Autodesk Inventor part; units mm, degrees
ref_plane "YZ Plane" through (0, 0, 0) normal (1, 0, 0) x (0, 1, 0)
ref_plane "XZ Plane" through (0, 0, 0) normal (0, 1, 0) x (-1, 0, 0)
ref_plane "XY Plane" through (0, 0, 0) normal (0, 0, 1) x (1, 0, 0)
sketch "Sketch1" plane through (0, 0, 0) normal (0, 1, 0) x (-1, 0, 0)
  line L0 (-19.05, 19.05) -> (19.05, 19.05)
  line L1 (19.05, 19.05) -> (19.05, -19.05)
  line L2 (19.05, -19.05) -> (-19.05, -19.05)
  line L3 (-19.05, -19.05) -> (-19.05, 19.05)
  circle A0 centre (0, 0) radius 6.35
  circle A1 centre (0, 0) radius 19.05 construction
  circle A2 centre (0, 0) radius 9.779 construction
  line L4 (19.05, -19.05) -> (-19.05, 19.05) construction
  line L5 (19.05, 19.05) -> (-19.05, -19.05) construction
  circle A3 centre (0, -9.779) radius 1.778
  circle A4 centre (6.9148, -6.9148) radius 1.778
  circle A5 centre (-6.9148, -6.9148) radius 1.778
  circle A6 centre (-6.9148, 6.9148) radius 1.778
  circle A7 centre (0, 9.779) radius 1.778
  circle A8 centre (6.9148, 6.9148) radius 1.778
  circle A9 centre (-9.779, 0) radius 2.032
  circle A10 centre (9.779, 0) radius 2.032
  circle A11 centre (-13.4704, 13.4704) radius 1.778
  circle A12 centre (13.4704, 13.4704) radius 1.778
  circle A13 centre (13.4704, -13.4704) radius 1.778
  circle A14 centre (-13.4704, -13.4704) radius 1.778
  dimension "d5" = 19.558
  dimension "d0" = 19.05
  dimension "d1" = 38.1
  dimension "d2" = 38.1
  dimension "d3" = 19.05
  dimension "d4" = 12.7
  dimension "d6" = 3.556
  dimension "d7" = 3.556
  dimension "d8" = 3.556
  dimension "d9" = 3.556
  dimension "d10" = 3.556
  dimension "d11" = 3.556
  dimension "d12" = 4.064
  dimension "d13" = 4.064
  dimension "d14" = 3.556
  dimension "d15" = 3.556
  dimension "d16" = 3.556
  dimension "d17" = 3.556
extrude "Extrusion1" add sketch "Sketch1" along normal blind 2.286
sketch "Sketch2" plane through (-19.05, 0, -19.05) normal (-1, 0, 0) x (0, 0, 1)
  line L0 (38.1, 0) -> (0, 0)
  line L1 (38.1, 0) -> (38.1, 2.286)
  line L2 (0, 2.286) -> (38.1, 2.286)
  line L3 (0, 0) -> (0, 2.286)
  circle A0 centre (46.9646, 57.15) radius 6.35
  line L4 (46.9646, 57.15) -> (0, 10.1854) construction
  line L5 (46.9646, 57.15) -> (113.3826, 57.15) construction
  circle A1 centre (33.4942, 43.6796) radius 6.35
  circle A2 centre (20.0238, 30.2092) radius 6.35
  circle A3 centre (46.9646, 57.15) radius 9.779 construction
  circle A4 centre (46.9646, 57.15) radius 19.05 construction
  line L6 (42.4745, 52.6599) -> (60.435, 70.6204) construction
  line L7 (46.9646, 57.15) -> (60.4393, 57.15) construction
  line L8 (60.435, 43.6796) -> (33.4942, 70.6204) construction
  line L9 (46.9646, 57.15) -> (60.4393, 57.15) construction
  line L10 (27.9146, 57.15) -> (66.0146, 57.15) construction
  circle A5 centre (40.0498, 64.0648) radius 1.778
  circle A6 centre (46.9646, 66.929) radius 1.778
  circle A7 centre (37.1856, 57.15) radius 1.778
  circle A8 centre (46.9646, 47.371) radius 1.778
  circle A9 centre (53.8794, 50.2352) radius 1.778
  circle A10 centre (56.7436, 57.15) radius 1.778
  circle A11 centre (53.8794, 64.0648) radius 2.032
  circle A12 centre (40.0498, 50.2352) radius 2.032
  circle A13 centre (46.9646, 76.2) radius 1.778
  circle A14 centre (27.9146, 57.15) radius 1.778
  circle A15 centre (46.9646, 38.1) radius 1.778
  circle A16 centre (66.0146, 57.15) radius 1.778
  point P0 (19.05, 0)
  dimension "d20" = 12.7
  dimension "d28" = 19.558
  dimension "d29" = 38.1
  dimension "d21" = 57.15
  dimension "d22" = 46.9646
  dimension "d23" = 135
  dimension "d24" = 12.7
  dimension "d25" = 19.05
  dimension "d26" = 12.7
  dimension "d27" = 19.05
  dimension "d30" = 45
  dimension "d31" = 135
  dimension "d32" = 3.556
  dimension "d33" = 3.556
  dimension "d34" = 3.556
  dimension "d35" = 3.556
  dimension "d36" = 3.556
  dimension "d37" = 3.556
  dimension "d38" = 4.064
  dimension "d39" = 4.064
  dimension "d40" = 3.556
  dimension "d41" = 3.556
  dimension "d42" = 3.556
  dimension "d43" = 3.556
properties part number "Channel Bracket B"
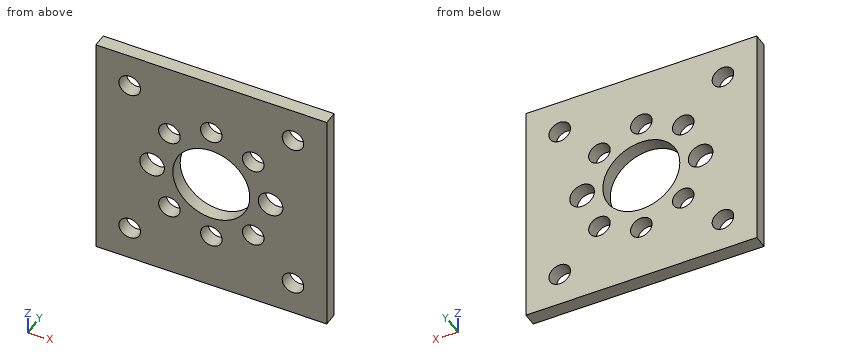
Part model, mm, in its own coordinate system. Give positions to 0.01 mm unless a question says otherwise; leave off trailing zeros. Order: outer loops, then holes, each group sorted by start corner. A loop starts at its lowest first (then second) coordinate and runs counter-clockwise, first axis right, second up. Notation, with made-up numbers: (47.5, 14.5) - (64.5, 14.5) arc R27 ccw to (64.5, 43.5) - close; hole circle Ø9 at (-7, 87). An arc over 180 degrees is marked (long way). Use a Markdown table: item, result.
1) Probe L1, parallel to Z at x = 0, y = 1.8; L2, parallel to X at y = 1.3, z = -13.5; L3, parallel to Z at x = -14.5, y = 1.2. List the from-to ranges inside material, lowest first. Write a range as from..to.
Checked values:
| item | result |
|---|---|
| L1 | -19.05..-11.56, -8..-6.35, 6.35..8, 11.56..19.05 |
| L2 | -19.05..-15.25, -11.69..11.69, 15.25..19.05 |
| L3 | -19.05..-14.92, -12.02..12.02, 14.92..19.05 |
2) Saw through at B-B on z = 0. List the corners of the cut face in (x, y).
Checked values:
| item | result |
|---|---|
| outline | (-19.05, 0) - (-11.81, 0) - (-11.81, 2.29) - (-19.05, 2.29) - close; (-7.75, 0) - (-6.35, 0) - (-6.35, 2.29) - (-7.75, 2.29) - close; (6.35, 0) - (7.75, 0) - (7.75, 2.29) - (6.35, 2.29) - close; (11.81, 0) - (19.05, 0) - (19.05, 2.29) - (11.81, 2.29) - close |
3) Saw through at C-C on y = 0.5. Count the separate pieces of the cut face and the enclosed holes in it, plus the area to 3 significant figures.
Checked values:
| item | result |
|---|---|
| separate pieces | 1 |
| enclosed holes | 13 |
| area | 1,200 mm² |
4) Saw through at A-A on x = 0. List the corners of the cut face in (y, z).
Checked values:
| item | result |
|---|---|
| outline | (0, -19.05) - (2.29, -19.05) - (2.29, -11.56) - (0, -11.56) - close; (0, -8) - (2.29, -8) - (2.29, -6.35) - (0, -6.35) - close; (0, 6.35) - (2.29, 6.35) - (2.29, 8) - (0, 8) - close; (0, 11.56) - (2.29, 11.56) - (2.29, 19.05) - (0, 19.05) - close |
5) Saw through at D-D on x = 4.5. List the corners of the cut face in (y, z).
Checked values:
| item | result |
|---|---|
| outline | (0, -19.05) - (2.29, -19.05) - (2.29, -4.48) - (0, -4.48) - close; (0, 4.48) - (2.29, 4.48) - (2.29, 19.05) - (0, 19.05) - close |
